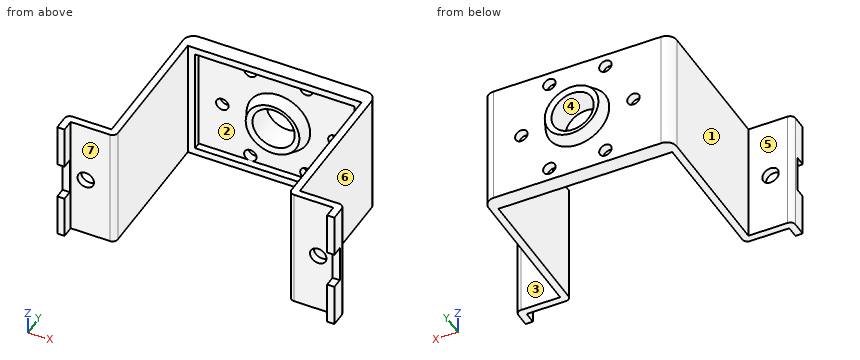
from build123d import *

# Parameters (mm, degrees)
SKETCH1_R                       = 7.7978
SKETCH1_R_2                     = 6.57225
SKETCH1_R_3                     = 5.17525
BOSS_EXTRUDE1_DEPTH             = 2.032
BOSS_EXTRUDE2_REACH             = 17.062
BOSS_EXTRUDE2_DIRECTION_2_REACH = 17.062
SKETCH4_W                       = 3.302
SKETCH4_H                       = 2.032
BOSS_EXTRUDE3_DEPTH             = 30.1244
FILLET1_R                       = 2.54
FILLET2_R                       = 2.54
SKETCH5_W                       = 9.0678
SKETCH5_H                       = 2.54
CUT_EXTRUDE1_DEPTH              = 116.84
SKETCH6_R                       = 2.01295
CUT_EXTRUDE2_DEPTH              = 5.7117
SKETCH7_R                       = 1.524
CUT_EXTRUDE3_DEPTH              = 42.5417
SKETCH9_W                       = 42.5577
SKETCH9_H                       = 30.1244
SKETCH9_W_2                     = 39.0017
SKETCH9_H_2                     = 26.5684
BOSS_EXTRUDE4_DEPTH             = 1.778


with BuildPart() as part:
    # Sketch1 → Boss-Extrude1 (new body)
    with BuildSketch(Plane(origin=(0, 0, 0), x_dir=(1, 0, 0), z_dir=(0, 1, 0))):
        with BuildLine():
            ThreePointArc((-23.05685, 9.9822), (-21.568952448, 13.574302448), (-17.97685, 15.0622))
            Line((-17.97685, 15.0622), (17.97685, 15.0622))
            ThreePointArc((17.97685, 15.0622), (21.568952448, 13.574302448), (23.05685, 9.9822))
            Line((23.05685, 9.9822), (23.05685, -9.9822))
            ThreePointArc((23.05685, -9.9822), (21.568952448, -13.574302448), (17.97685, -15.0622))
            Line((17.97685, -15.0622), (-17.97685, -15.0622))
            ThreePointArc((-17.97685, -15.0622), (-21.568952448, -13.574302448), (-23.05685, -9.9822))
            Line((-23.05685, -9.9822), (-23.05685, 9.9822))
        make_face()
        Circle(SKETCH1_R, mode=Mode.SUBTRACT)
        Circle(SKETCH1_R)
        Circle(SKETCH1_R_2, mode=Mode.SUBTRACT)
        Circle(SKETCH1_R_2)
        Circle(SKETCH1_R_3, mode=Mode.SUBTRACT)
    extrude(amount=-BOSS_EXTRUDE1_DEPTH)

    # Sketch2 → Revolve1 (revolve)
    with BuildSketch(Plane(origin=(0, 0, 0), x_dir=(0, 0, -1), z_dir=(1, 0, 0))):
        Polygon((-5.17525, 2.286), (-6.57225, 2.794), (-7.7978, 0), (-5.17525, 0), align=None)
    revolve1 = revolve(axis=Axis((0, 0, 0), (0, 1, 0)))

    # Boss-Extrude2: up to this face of the body (flat: up to its plane)
    boss_extrude2_end = Plane(part.part.faces().sort_by_distance((0, -1.016, 15.0622))[0])
    # Sketch3 → Boss-Extrude2 (add, up to the picked face)
    with BuildSketch(Plane.XY, mode=Mode.PRIVATE) as boss_extrude2_sk1:
        with BuildLine():
            ThreePointArc((-23.05685, -1.27), (-22.684875612, -0.371974388), (-21.78685, 0))
            Line((-21.78685, 0), (-21.27885, 0))
            Line((-21.27885, 0), (-21.27885, -37.338))
            ThreePointArc((-21.27885, -37.338), (-21.650824388, -38.236025612), (-22.54885, -38.608))
            Line((-22.54885, -38.608), (-23.05685, -38.608))
            Line((-23.05685, -38.608), (-32.16275, -38.608))
            Line((-32.16275, -38.608), (-32.16275, -41.5417))
            Line((-32.16275, -41.5417), (-33.94075, -41.5417))
            Line((-33.94075, -41.5417), (-33.94075, -38.1))
            ThreePointArc((-33.94075, -38.1), (-33.568775612, -37.201974388), (-32.67075, -36.83))
            Line((-32.67075, -36.83), (-32.16275, -36.83))
            Line((-32.16275, -36.83), (-23.05685, -36.83))
            Line((-23.05685, -36.83), (-23.05685, -1.27))
        make_face()
    boss_extrude2_tool1 = split(extrude(boss_extrude2_sk1.sketch, amount=BOSS_EXTRUDE2_REACH, mode=Mode.PRIVATE), bisect_by=boss_extrude2_end, keep=Keep.BOTH, mode=Mode.PRIVATE)
    add(boss_extrude2_tool1.solids().sort_by_distance((-32.41675, -37.264285, 0))[0])
    # Sketch3 → Boss-Extrude2 (add, up to the picked face)
    with BuildSketch(Plane.XY, mode=Mode.PRIVATE) as boss_extrude2_sk2:
        with BuildLine():
            Line((21.27885, 0), (21.27885, -37.338))
            ThreePointArc((21.27885, -37.338), (21.650824388, -38.236025612), (22.54885, -38.608))
            Line((22.54885, -38.608), (23.05685, -38.608))
            Line((23.05685, -38.608), (32.16275, -38.608))
            Line((32.16275, -38.608), (32.16275, -41.5417))
            Line((32.16275, -41.5417), (33.94075, -41.5417))
            Line((33.94075, -41.5417), (33.94075, -38.1))
            ThreePointArc((33.94075, -38.1), (33.568775612, -37.201974388), (32.67075, -36.83))
            Line((32.67075, -36.83), (32.16275, -36.83))
            Line((32.16275, -36.83), (23.05685, -36.83))
            Line((23.05685, -36.83), (23.05685, -1.27))
            ThreePointArc((23.05685, -1.27), (22.684875612, -0.371974388), (21.78685, 0))
            Line((21.78685, 0), (21.27885, 0))
        make_face()
    boss_extrude2_tool2 = split(extrude(boss_extrude2_sk2.sketch, amount=BOSS_EXTRUDE2_REACH, mode=Mode.PRIVATE), bisect_by=boss_extrude2_end, keep=Keep.BOTH, mode=Mode.PRIVATE)
    add(boss_extrude2_tool2.solids().sort_by_distance((27.6098, -38.173715, 0))[0])

    # Boss-Extrude2 direction 2: up to this face of the body (flat: up to its plane)
    boss_extrude2_direction_2_end = Plane(part.part.faces().sort_by_distance((0, -1.016, -15.0622))[0])
    # Sketch3 → Boss-Extrude2 direction 2 (add, up to the picked face)
    with BuildSketch(Plane.XY, mode=Mode.PRIVATE) as boss_extrude2_direction_2_sk1:
        with BuildLine():
            ThreePointArc((-23.05685, -1.27), (-22.684875612, -0.371974388), (-21.78685, 0))
            Line((-21.78685, 0), (-21.27885, 0))
            Line((-21.27885, 0), (-21.27885, -37.338))
            ThreePointArc((-21.27885, -37.338), (-21.650824388, -38.236025612), (-22.54885, -38.608))
            Line((-22.54885, -38.608), (-23.05685, -38.608))
            Line((-23.05685, -38.608), (-32.16275, -38.608))
            Line((-32.16275, -38.608), (-32.16275, -41.5417))
            Line((-32.16275, -41.5417), (-33.94075, -41.5417))
            Line((-33.94075, -41.5417), (-33.94075, -38.1))
            ThreePointArc((-33.94075, -38.1), (-33.568775612, -37.201974388), (-32.67075, -36.83))
            Line((-32.67075, -36.83), (-32.16275, -36.83))
            Line((-32.16275, -36.83), (-23.05685, -36.83))
            Line((-23.05685, -36.83), (-23.05685, -1.27))
        make_face()
    boss_extrude2_direction_2_tool1 = split(extrude(boss_extrude2_direction_2_sk1.sketch, amount=-BOSS_EXTRUDE2_DIRECTION_2_REACH, mode=Mode.PRIVATE), bisect_by=boss_extrude2_direction_2_end, keep=Keep.BOTH, mode=Mode.PRIVATE)
    add(boss_extrude2_direction_2_tool1.solids().sort_by_distance((-32.41675, -37.264285, 0))[0])
    # Sketch3 → Boss-Extrude2 direction 2 (add, up to the picked face)
    with BuildSketch(Plane.XY, mode=Mode.PRIVATE) as boss_extrude2_direction_2_sk2:
        with BuildLine():
            Line((21.27885, 0), (21.27885, -37.338))
            ThreePointArc((21.27885, -37.338), (21.650824388, -38.236025612), (22.54885, -38.608))
            Line((22.54885, -38.608), (23.05685, -38.608))
            Line((23.05685, -38.608), (32.16275, -38.608))
            Line((32.16275, -38.608), (32.16275, -41.5417))
            Line((32.16275, -41.5417), (33.94075, -41.5417))
            Line((33.94075, -41.5417), (33.94075, -38.1))
            ThreePointArc((33.94075, -38.1), (33.568775612, -37.201974388), (32.67075, -36.83))
            Line((32.67075, -36.83), (32.16275, -36.83))
            Line((32.16275, -36.83), (23.05685, -36.83))
            Line((23.05685, -36.83), (23.05685, -1.27))
            ThreePointArc((23.05685, -1.27), (22.684875612, -0.371974388), (21.78685, 0))
            Line((21.78685, 0), (21.27885, 0))
        make_face()
    boss_extrude2_direction_2_tool2 = split(extrude(boss_extrude2_direction_2_sk2.sketch, amount=-BOSS_EXTRUDE2_DIRECTION_2_REACH, mode=Mode.PRIVATE), bisect_by=boss_extrude2_direction_2_end, keep=Keep.BOTH, mode=Mode.PRIVATE)
    add(boss_extrude2_direction_2_tool2.solids().sort_by_distance((27.6098, -38.173715, 0))[0])

    # Sketch4 → Boss-Extrude3 (add)
    with BuildSketch(Plane.XY.offset(15.0622)):
        with BuildLine():
            ThreePointArc((-23.05685, -1.27), (-22.684875612, -0.371974388), (-21.78685, 0))
            Line((-21.78685, 0), (-23.05685, 0))
            Line((-23.05685, 0), (-23.05685, -1.27))
        make_face()
        with BuildLine():
            Line((-21.27885, -2.032), (-21.27885, 0))
            Line((-21.27885, 0), (-21.78685, 0))
            ThreePointArc((-21.78685, 0), (-22.684875612, -0.371974388), (-23.05685, -1.27))
            Line((-23.05685, -1.27), (-23.05685, -2.032))
            Line((-23.05685, -2.032), (-21.27885, -2.032))
        make_face()
        with Locations((-19.62785, -1.016)):
            Rectangle(SKETCH4_W, SKETCH4_H)
        Polygon((23.05685, 0), (21.27885, 0), (17.97685, 0), (17.97685, -2.032), (21.27885, -2.032), (23.05685, -2.032), align=None)
    extrude(amount=-BOSS_EXTRUDE3_DEPTH)

    # Fillet1
    fillet1_edges = [part.edges().sort_by_distance(p)[0] for p in [
        (23.05685, 0, 0),
    ]]
    fillet(fillet1_edges, radius=FILLET1_R)

    # Fillet2
    fillet2_edges = [part.edges().sort_by_distance(p)[0] for p in [
        (-23.05685, 0, 0),
    ]]
    fillet(fillet2_edges, radius=FILLET2_R)

    # Sketch5 → Cut-Extrude1 (cut)
    with BuildSketch(Plane.ZY.offset(33.94075)):
        with Locations((0, -40.2717)):
            Rectangle(SKETCH5_W, SKETCH5_H)
    extrude(amount=-CUT_EXTRUDE1_DEPTH, mode=Mode.SUBTRACT)

    # Sketch6 → Cut-Extrude2 (cut, through all)
    with BuildSketch(Plane(origin=(0, -36.83, 0), x_dir=(1, 0, 0), z_dir=(0, 1, 0))):
        with Locations((-28.4734, 0)):
            Circle(SKETCH6_R)
        with Locations((28.4734, 0)):
            Circle(SKETCH6_R)
    extrude(amount=-CUT_EXTRUDE2_DEPTH, mode=Mode.SUBTRACT)

    # Sketch7 → Cut-Extrude3 (cut, through all)
    with BuildSketch(Plane(origin=(0, 0, 0), x_dir=(1, 0, 0), z_dir=(0, 1, 0))):
        with Locations((13.725830849, 0)):
            Circle(SKETCH7_R)
        with Locations((-13.725830849, 0)):
            Circle(SKETCH7_R)
        with Locations((-6.862915424, -11.886918203)):
            Circle(SKETCH7_R)
        with Locations((6.862915424, 11.886918203)):
            Circle(SKETCH7_R)
        with Locations((-6.862915424, 11.886918203)):
            Circle(SKETCH7_R)
        with Locations((6.862915424, -11.886918203)):
            Circle(SKETCH7_R)
    extrude(amount=-CUT_EXTRUDE3_DEPTH, mode=Mode.SUBTRACT)

    # Mirror4: Revolve1 across plane
    add(revolve1.mirror(Plane.ZX.offset(-1.016)))

    # Sketch9 → Boss-Extrude4 (add)
    with BuildSketch(Plane.XZ.offset(2.032)):
        Rectangle(SKETCH9_W, SKETCH9_H)
        Rectangle(SKETCH9_W_2, SKETCH9_H_2, mode=Mode.SUBTRACT)
    extrude(amount=BOSS_EXTRUDE4_DEPTH)


solid = part.part
CAD build for the part. Positions are in the model's coordinates, mm. Face numbers are marked on the shaded views. A direction names the side the tool comes from. Round coordinates to 2 decimals unless told otherwise and drop trailing zeros. Write each loop counter-clockwise with the first axis right and the second up, starting at its lowest first coordinate (ties: lowest second). Pieces come first, ordered by that corner, then holes. Notation, with made-up numbers: (31.25, 23.25) -> (79.25, 23.25) arc R37 cw to (79.25, 61.25) -> close; hole circle Ø2 at (67.25, 70.5). An arc over 180 degrees is marked (long way). Answer as a JSON object with one key per item and string values.
(1) Pin check, flat tips, straight feed: P1, Ø6, axis at x = 0, z = 0, coming from the -Y side; P2, Ø15, axis at y = -20.5, z = 6.5, coming from the -X side; P3, Ø3.5, axis at x = 13.73, z = 0, coming from the +Y side; P4, Ø2, axis at x = -23.5, z = -10, coming from the +Y side. Stop position of each tip, or through.
Reported:
{"P1": "passes through", "P2": "stops at x = -23.06", "P3": "stops at y = 0", "P4": "stops at y = -0.95"}
(2) Which spindle directions (+Z, -Z, +X, -X, +Y, -Y) get a long thin tool onto all of the face, cutting with end or side? Do the marked faces 4, 5, 6 and 7. Say none if no direction does.
Reported:
{"face 4": "+Y, -Y", "face 5": "+Z, -Z, -X, +Y", "face 6": "+Z, -Z, +X, +Y", "face 7": "+Z, -Z, -Y"}
(3) Two-plate mould, pull along X, no slides. Class the marked faces 1, 2 and 3: +X half, -X half, draft (parallel to the pull), parting line (faces both ways), or undercut.
Reported:
{"face 1": "-X half", "face 2": "undercut", "face 3": "draft"}
(4) Band-saw the part on C-C, the plane z = 0. Count the separate pieces of the cut face and the enclosed holes in it, then the cut area to 3 significant figures.
Reported:
{"separate pieces": "6", "enclosed holes": "0", "area": "239 mm^2"}
(5) Band-saw the part on A-A, the plane x = 0. List the corners of the cut face in (y, z).
Reported:
{"outline": "(-4.83, -6.57) -> (-2.03, -7.8) -> (-2.03, -13.28) -> (-3.81, -13.28) -> (-3.81, -15.06) -> (0, -15.06) -> (0, -7.8) -> (2.79, -6.57) -> (2.29, -5.18) -> (-4.32, -5.18) -> close; (-4.83, 6.57) -> (-4.32, 5.18) -> (2.29, 5.18) -> (2.79, 6.57) -> (0, 7.8) -> (0, 15.06) -> (-3.81, 15.06) -> (-3.81, 13.28) -> (-2.03, 13.28) -> (-2.03, 7.8) -> close"}
(6) Band-saw the part on B-B, the plane y = -11. List the corners of the cut face in (x, z).
Reported:
{"outline": "(-23.06, -15.06) -> (-21.28, -15.06) -> (-21.28, 15.06) -> (-23.06, 15.06) -> close; (21.28, -15.06) -> (23.06, -15.06) -> (23.06, 15.06) -> (21.28, 15.06) -> close"}
(7) Band-saw the part on D-D, the plane x = -10.5. List the corners of the cut face in (y, z).
Reported:
{"outline": "(-3.81, -15.06) -> (0, -15.06) -> (0, 15.06) -> (-3.81, 15.06) -> (-3.81, 13.28) -> (-2.03, 13.28) -> (-2.03, -13.28) -> (-3.81, -13.28) -> close"}
(8) Probe probe 1 along X at (y, z) = (-29.5, 6); probe 2 along Y at (x, z) = (20.5, 7.5); probe 3 along Y at (x, z) = (-24.5, -8). List the from-to ranges inside material, lowest first. Write a range as [from, to].
Reported:
{"probe 1": "x = [-23.06, -21.28], [21.28, 23.06]", "probe 2": "y = [-3.81, 0]", "probe 3": "y = [-38.61, -36.83]"}
